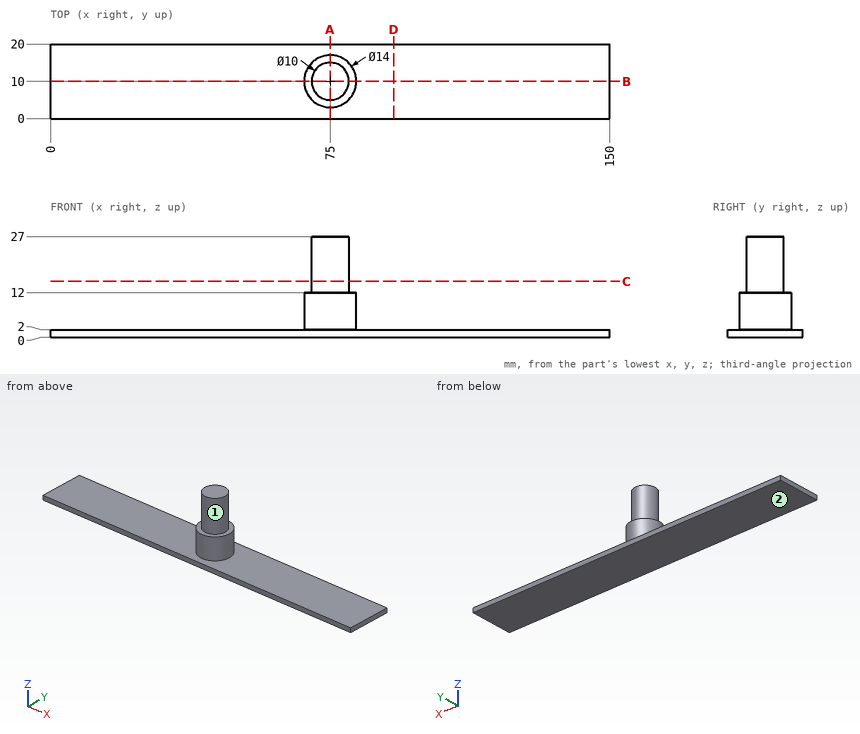
Design review of the part shown in the three views and the two pictorial views. Dimensions are in mm from the part's minimum x, y and z. A direction names the side the tool comes from. Give positions to 0.01 mm unless a question says otherwise; leave off trailing zeros. Write each loop counter-clockwise with the first axis right and the second up, starting at its lowest first coordinate (ties: lowest second). Pieces come first, ordered by that corner, then holes. Notation, with made-up numbers: M 79.25,65.25 L 95.25,65.25 A35 ccw 95.25,99.25 Z; hole C 66,60 d10. An arc over 180 degrees is marked long. Answer in a Markdown table with one row per item.
Item 1: For P1, Ø1.5, axis at y = 9.5, z = 5.5, coming from the -X side; P2, Ø1.5, axis at y = 12.5, z = 9.5, coming from the +X side; P3, Ø1.5, axis at y = 13, z = 21.5, coming from the +X side, all flat-tipped, find the tip position at first contact; note any pin that passes through.
Check sheet entries:
| item | result |
|---|---|
| P1 | x = 68 |
| P2 | x = 81.78 |
| P3 | x = 79.47 |
Item 2: Add section C-C on z = 15. Give the boundary of the cut face in (x, y), plus the area to 3 significant figures.
Check sheet entries:
| item | result |
|---|---|
| outline | C 75,10 d10 |
| area | 78.5 mm2 |
Item 3: Add section A-A on x = 75. Give the boundary of the cut face in (y, z), plus the area to 3 significant figures.
Check sheet entries:
| item | result |
|---|---|
| outline | M 0,0 L 20,0 L 20,2 L 17,2 L 17,12 L 15,12 L 15,27 L 5,27 L 5,12 L 3,12 L 3,2 L 0,2 Z |
| area | 330 mm2 |
Item 4: Tool access review of the marked faces 1 and 2: name each direction out of +Z, -Z, +X, -X, +Y, -Y from which nothing blocks a thin tool from reaching the whole face with its end or side.
Check sheet entries:
| item | result |
|---|---|
| face 1 | +Z |
| face 2 | -Z, +X, -X, +Y, -Y |
Item 5: For line 1 along Z through (x, y) = (96.5, 16.5); line 2 along Z through (x, y) = (76, 5); line 3 along X through (y, z) = (6, 21.5), list the stretches that pass through material, from the lowest coordinate up.
Check sheet entries:
| item | result |
|---|---|
| line 1 | 0 to 2 |
| line 2 | 0 to 12 |
| line 3 | 72 to 78 |
Item 6: Add section D-D on x = 92. Give the boundary of the cut face in (y, z).
Check sheet entries:
| item | result |
|---|---|
| outline | M 0,0 L 20,0 L 20,2 L 0,2 Z |
Item 7: Add section B-B on y = 10. Give the boundary of the cut face in (x, z).
Check sheet entries:
| item | result |
|---|---|
| outline | M 0,0 L 150,0 L 150,2 L 82,2 L 82,12 L 80,12 L 80,27 L 70,27 L 70,12 L 68,12 L 68,2 L 0,2 Z |
